Input: part model. Units: mm. Frame: model coordinates. A direction names the side the tool comes from. Coordinates: 2 decimals unless noted, no trailing zeros. Write each loop counter-clockwise with the first axis right and the second up, starting at its lowest first coordinate (ties: lowest second). Pieces come first, ordered by that corner, then holes. Notation, with made-up numbers: (77, 62) - (101, 62) arc R8 ccw to (101, 74) - close; hole circle Ø1 at (-30, -18). An arc over 180 degrees is marked (long way). Use a Markdown table: item, result. Add a question column.
Q1. Material intervals for probe 1 along X at (y, z) = (795.5, 0); probe 2 along Y at (x, z) = (74.5, -541); probe 3 along Z at (x, y) = (34, 302), sorted ascending. Write a range as from..to.
Q2. Section query C-C (x = 410). Return the cut outline in (y, z), then the cut area to 3 significant figures.
Q3. Set-up query: faces 1 (the face through (21.984, 503.14, -499.516)), 2 (the face through (19.786, 9.86, -449.565)). Return all of +Z, -Z, +X, -X, +Y, -Y with unobstructed straight access to the full face (end or side cutting, diameter ignored); none if empty.
Q4. Pin query (flat end, axial travel): P1, Ø1, axis at x = -248, z = 522.5, coming from the +Y side; P2, Ø17.5, axis at x = 441.94, z = -441.94, coming from the +Y side; P3, Ø1.5, axis at y = 808, z = 305, coming from the -X side; P4, Ø5, axis at x = 40.5, y = 223, coming from the +Z side. Return the tip coordinate at first contact, or that it passes through.
Q5. Mould query, pull axis X, two halves, no side actions, for faces 3 (the face through (165, 20, -476)), 4 (the face through (694.043, 9.86, -91.126)), 5 (the face through (-428, 20, 141)). Classes: released by +X, released by -X, zero draft, split by the parting line, or undercut.
Q6. Section query B-B (z = 62.5). Return the cut outline in (x, y).
Q7. Section query A-A (y = 874.5). Return the cut outline in (x, z), then the cut area to 3 significant figures.
from build123d import *

# Parameters (mm, degrees)
SKETCH1_R           = 500
SKETCH1_R_2         = 484
BOSS_EXTRUDE1_DEPTH = 1000
SKETCH2_R           = 700
SKETCH2_R_2         = 450
SKETCH2_R_3         = 11
BOSS_EXTRUDE2_DEPTH = 20


with BuildPart() as part:
    # Sketch1 → Boss-Extrude1 (new body)
    with BuildSketch(Plane(origin=(0, 0, 0), x_dir=(1, 0, 0), z_dir=(0, 1, 0))):
        with Locations(Location((0, 0, 0), (0, 0, 270))):
            Circle(SKETCH1_R)
        with Locations(Location((0, 0, 0), (0, 0, 270))):
            Circle(SKETCH1_R_2, mode=Mode.SUBTRACT)
    extrude(amount=BOSS_EXTRUDE1_DEPTH)

    # Sketch2 → Boss-Extrude2 (add)
    with BuildSketch(Plane(origin=(0, 0, 0), x_dir=(1, 0, 0), z_dir=(0, 1, 0))):
        with Locations(Location((0, 0, 0), (0, 0, 270))):
            Circle(SKETCH2_R)
        with Locations(Location((0, 0, 0), (0, 0, 270))):
            Circle(SKETCH2_R_2, mode=Mode.SUBTRACT)
        with Locations(Location((0, 625, 0), (0, 0, 270))):
            Circle(SKETCH2_R_3, mode=Mode.SUBTRACT)
        with Locations(Location((121.93145126, 612.990800252, 0), (0, 0, 270))):
            Circle(SKETCH2_R_3, mode=Mode.SUBTRACT)
        with Locations(Location((239.177145228, 577.42470782, 0), (0, 0, 270))):
            Circle(SKETCH2_R_3, mode=Mode.SUBTRACT)
        with Locations(Location((347.231395637, 519.668507689, 0), (0, 0, 270))):
            Circle(SKETCH2_R_3, mode=Mode.SUBTRACT)
        with Locations(Location((441.941738242, 441.941738242, 0), (0, 0, 270))):
            Circle(SKETCH2_R_3, mode=Mode.SUBTRACT)
        with Locations(Location((519.668507689, 347.231395637, 0), (0, 0, 270))):
            Circle(SKETCH2_R_3, mode=Mode.SUBTRACT)
        with Locations(Location((577.42470782, 239.177145228, 0), (0, 0, 270))):
            Circle(SKETCH2_R_3, mode=Mode.SUBTRACT)
        with Locations(Location((612.990800252, 121.93145126, 0), (0, 0, 270))):
            Circle(SKETCH2_R_3, mode=Mode.SUBTRACT)
        with Locations(Location((625, 0, 0), (0, 0, 270))):
            Circle(SKETCH2_R_3, mode=Mode.SUBTRACT)
        with Locations(Location((612.990800252, -121.93145126, 0), (0, 0, 270))):
            Circle(SKETCH2_R_3, mode=Mode.SUBTRACT)
        with Locations(Location((577.42470782, -239.177145228, 0), (0, 0, 270))):
            Circle(SKETCH2_R_3, mode=Mode.SUBTRACT)
        with Locations(Location((519.668507689, -347.231395637, 0), (0, 0, 270))):
            Circle(SKETCH2_R_3, mode=Mode.SUBTRACT)
        with Locations(Location((441.941738242, -441.941738242, 0), (0, 0, 270))):
            Circle(SKETCH2_R_3, mode=Mode.SUBTRACT)
        with Locations(Location((347.231395637, -519.668507689, 0), (0, 0, 270))):
            Circle(SKETCH2_R_3, mode=Mode.SUBTRACT)
        with Locations(Location((239.177145228, -577.42470782, 0), (0, 0, 270))):
            Circle(SKETCH2_R_3, mode=Mode.SUBTRACT)
        with Locations(Location((121.93145126, -612.990800252, 0), (0, 0, 270))):
            Circle(SKETCH2_R_3, mode=Mode.SUBTRACT)
        with Locations(Location((0, -625, 0), (0, 0, 270))):
            Circle(SKETCH2_R_3, mode=Mode.SUBTRACT)
        with Locations(Location((-121.93145126, -612.990800252, 0), (0, 0, 270))):
            Circle(SKETCH2_R_3, mode=Mode.SUBTRACT)
        with Locations(Location((-239.177145228, -577.42470782, 0), (0, 0, 270))):
            Circle(SKETCH2_R_3, mode=Mode.SUBTRACT)
        with Locations(Location((-347.231395637, -519.668507689, 0), (0, 0, 270))):
            Circle(SKETCH2_R_3, mode=Mode.SUBTRACT)
        with Locations(Location((-441.941738242, -441.941738242, 0), (0, 0, 270))):
            Circle(SKETCH2_R_3, mode=Mode.SUBTRACT)
        with Locations(Location((-519.668507689, -347.231395637, 0), (0, 0, 270))):
            Circle(SKETCH2_R_3, mode=Mode.SUBTRACT)
        with Locations(Location((-577.42470782, -239.177145228, 0), (0, 0, 270))):
            Circle(SKETCH2_R_3, mode=Mode.SUBTRACT)
        with Locations(Location((-612.990800252, -121.93145126, 0), (0, 0, 270))):
            Circle(SKETCH2_R_3, mode=Mode.SUBTRACT)
        with Locations(Location((-625, 0, 0), (0, 0, 270))):
            Circle(SKETCH2_R_3, mode=Mode.SUBTRACT)
        with Locations(Location((-612.990800252, 121.93145126, 0), (0, 0, 270))):
            Circle(SKETCH2_R_3, mode=Mode.SUBTRACT)
        with Locations(Location((-577.42470782, 239.177145228, 0), (0, 0, 270))):
            Circle(SKETCH2_R_3, mode=Mode.SUBTRACT)
        with Locations(Location((-519.668507689, 347.231395637, 0), (0, 0, 270))):
            Circle(SKETCH2_R_3, mode=Mode.SUBTRACT)
        with Locations(Location((-441.941738242, 441.941738242, 0), (0, 0, 270))):
            Circle(SKETCH2_R_3, mode=Mode.SUBTRACT)
        with Locations(Location((-347.231395637, 519.668507689, 0), (0, 0, 270))):
            Circle(SKETCH2_R_3, mode=Mode.SUBTRACT)
        with Locations(Location((-239.177145228, 577.42470782, 0), (0, 0, 270))):
            Circle(SKETCH2_R_3, mode=Mode.SUBTRACT)
        with Locations(Location((-121.93145126, 612.990800252, 0), (0, 0, 270))):
            Circle(SKETCH2_R_3, mode=Mode.SUBTRACT)
    extrude(amount=BOSS_EXTRUDE2_DEPTH)


solid = part.part
Values follow:
| question | item | result |
|---|---|---|
| 1 | probe 1 | -500..-484, 484..500 |
| 1 | probe 2 | 0..20 |
| 1 | probe 3 | -498.84..-482.8, 482.8..498.84 |
| 2 | outline | (0, -567.36) - (20, -567.36) - (20, -286.18) - (1000, -286.18) - (1000, -257.21) - (20, -257.21) - (20, -185.47) - (0, -185.47) - close; (0, 185.47) - (20, 185.47) - (20, 257.21) - (1000, 257.21) - (1000, 286.18) - (20, 286.18) - (20, 567.36) - (0, 567.36) - close |
| 2 | area | 72,100 mm2 |
| 3 | face 1 | +Y |
| 3 | face 2 | +Y, -Y |
| 4 | P1 | y = 20 |
| 4 | P2 | through |
| 4 | P3 | x = -396.78 |
| 4 | P4 | z = 498.55 |
| 5 | face 3 | zero draft |
| 5 | face 4 | split by the parting line |
| 5 | face 5 | undercut |
| 6 | outline | (-697.2, 0) - (-445.64, 0) - (-445.64, 20) - (-479.95, 20) - (-479.95, 1000) - (-496.08, 1000) - (-496.08, 20) - (-697.2, 20) - close; (445.64, 0) - (697.2, 0) - (697.2, 20) - (496.08, 20) - (496.08, 1000) - (479.95, 1000) - (479.95, 20) - (445.64, 20) - close |
| 7 | outline | circle Ø1000 at (0, 0); hole circle Ø968 at (0, 0) |
| 7 | area | 49,500 mm2 |
